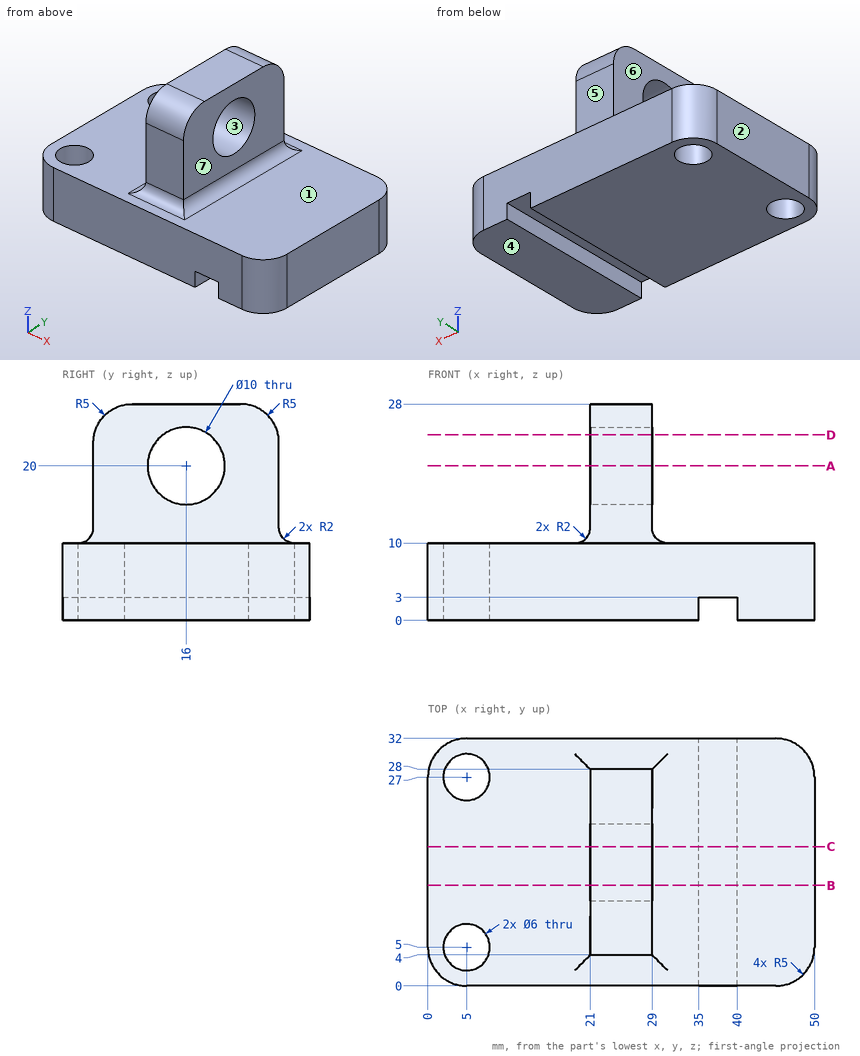
Can you work these out from the drawing? Everything is in mm from the part's minimum corner. A direction names the side the tool comes from. Round coordinates to 2 decimals unless told otherwise and drop trailing zeros. Order: outer loops, then holes, each group sorted by start corner. A loop starts at its lowest first (then second) coordinate and runs counter-clockwise, first axis right, second up. Notation, with made-up numbers: (6, 54) - (16, 54) arc R31 cw to (16, 81) - close; hole circle Ø4 at (1.5, 7). An arc over 180 degrees is marked (long way). Answer in a Markdown table with one row per item.
(1) For P1, Ø5.5, axis at x = 5, y = 5, coming from the +Z side (3 decimals); P2, Ø8, axis at y = 21.5, z = 18.5, coming from the +X side; P3, Ø4, axis at x = 24.5, z = 19, coming from the -Y side; P4, Ø4, axis at x = 22.5, z = 21, coming from the +Y side, each with a flat end and sliding along its axis, tell me the tip position at first contact or that it passes through.
From the geometry:
| item | result |
|---|---|
| P1 | passes through |
| P2 | stops at x = 29 |
| P3 | stops at y = 4 |
| P4 | stops at y = 28 |
(2) Suppose I cut it at C-C, the plane y = 18. Please give me the cut outline in (x, z).
From the geometry:
| item | result |
|---|---|
| outline | (0, 0) - (35, 0) - (35, 3) - (40, 3) - (40, 0) - (50, 0) - (50, 10) - (31, 10) arc R2 cw to (29, 12) - (29, 15.42) - (21, 15.42) - (21, 12) arc R2 cw to (19, 10) - (0, 10) - close; (21, 24.58) - (29, 24.58) - (29, 28) - (21, 28) - close |
(3) Suppose I cut it at D-D, the plane z = 24. Please give me the cut outline in (x, y).
From the geometry:
| item | result |
|---|---|
| outline | (21, 4.1) - (29, 4.1) - (29, 13) - (21, 13) - close; (21, 19) - (29, 19) - (29, 27.9) - (21, 27.9) - close |
(4) If we mould it in two halves opening along Z, with no side actions, what happens to the marked faces 1, 2, 3 and 4? For each: released by +Z, released by -Z, zero draft, split by the parting line, or undercut.
From the geometry:
| item | result |
|---|---|
| face 1 | released by +Z |
| face 2 | zero draft |
| face 3 | undercut |
| face 4 | released by -Z |
(5) Which directions (+Z, -Z, +X, -X, +Y, -Y) give clear straight access to the entire face, cutting with the end or side of a thin tool? Please do the marked faces 5, 6 and 7.
From the geometry:
| item | result |
|---|---|
| face 5 | +Z, +X, -X, +Y |
| face 6 | +Z, -X, +Y, -Y |
| face 7 | +Z, +X, +Y, -Y |
(6) Suppose I cut it at A-A, the plane z = 20. Please give me the cut outline in (x, y), plus the area to 3 significant figures.
From the geometry:
| item | result |
|---|---|
| outline | (21, 4) - (29, 4) - (29, 11) - (21, 11) - close; (21, 21) - (29, 21) - (29, 28) - (21, 28) - close |
| area | 112 mm2 |
(7) Suppose I cut it at B-B, the plane y = 13. Please give me the cut outline in (x, z).
From the geometry:
| item | result |
|---|---|
| outline | (0, 0) - (35, 0) - (35, 3) - (40, 3) - (40, 0) - (50, 0) - (50, 10) - (31, 10) arc R2 cw to (29, 12) - (29, 16) - (21, 16) - (21, 12) arc R2 cw to (19, 10) - (0, 10) - close; (21, 24) - (29, 24) - (29, 28) - (21, 28) - close |
(8) Please list where these lines run through material, in increasing order: L1, parallel to Y at x = 5, z = 7.5; L2, parallel to Y at x = 23.75, z = 20; L3, parallel to Z at x = 11, y = 9.5. Write a range as from..to.
From the geometry:
| item | result |
|---|---|
| L1 | y = 0..2, 8..24, 30..32 |
| L2 | y = 4..11, 21..28 |
| L3 | z = 0..10 |
